The listing builds one solid part. Answer for the finished solid, in the listing's coordinates (mm). A direction names the side the tool comes from. Round coordinates to 2 decimals unless told otherwise and drop trailing zeros. Order: outer loops, then holes, each group sorted by start corner. A loop starts at its lowest first (then second) coordinate and runs counter-clockwise, first axis right, second up. Notation, with made-up numbers: (57, 20.25) - (75, 20.25) arc R5 cw to (75, 29.25) - close; hole circle Ø1 at (-23, -32). An arc over 180 degrees is marked (long way). Write item = value, one per line.
from build123d import *

# Parameters (mm, degrees)
BOSS_EXTRUDE1_DEPTH       = 10.5
BOSS_EXTRUDE2_DEPTH       = 4.5
BOSS_EXTRUDE3_DEPTH       = 7
SKETCH4_W                 = 9.5
SKETCH4_H                 = 16
BOSS_EXTRUDE4_DEPTH       = 6
SKETCH5_W                 = 2.5
SKETCH5_H                 = 2
CUT_EXTRUDE1_DEPTH        = 26.5
SKETCH6_W                 = 6
SKETCH6_H                 = 15
CUT_EXTRUDE2_DEPTH        = 5.5
F_2_CLEARANCE_HOLE1_D     = 2.5
F_2_CLEARANCE_HOLE1_DEPTH = 22
CHAMFER1_SIZE             = 0.25


with BuildPart() as part:
    # Sketch1 → Boss-Extrude1 (new body)
    with BuildSketch(Plane(origin=(0, 0, 0), x_dir=(0, -1, 0), z_dir=(-1, 0, 0))):
        with BuildLine():
            Line((14.924811557, 17.5), (-14.924811557, 17.5))
            ThreePointArc((-14.924811557, 17.5), (-16.263455967, 16.263455967), (-17.5, 14.924811557))
            Line((-17.5, 14.924811557), (-17.5, -14.924811557))
            ThreePointArc((-17.5, -14.924811557), (-16.263455967, -16.263455967), (-14.924811557, -17.5))
            Line((-14.924811557, -17.5), (14.924811557, -17.5))
            ThreePointArc((14.924811557, -17.5), (16.263455967, -16.263455967), (17.5, -14.924811557))
            Line((17.5, -14.924811557), (17.5, 14.924811557))
            ThreePointArc((17.5, 14.924811557), (16.263455967, 16.263455967), (14.924811557, 17.5))
        make_face()
    extrude(amount=-BOSS_EXTRUDE1_DEPTH)

    # Sketch2 → Boss-Extrude2 (add)
    with BuildSketch(Plane(origin=(10.5, 0, 0), x_dir=(0, 0, -1), z_dir=(1, 0, 0))):
        with BuildLine():
            Line((-17.5, -11.608186766), (-17.5, 11.608186766))
            ThreePointArc((-17.5, 11.608186766), (-14.849242405, 14.849242405), (-11.608186766, 17.5))
            Line((-11.608186766, 17.5), (11.608186766, 17.5))
            ThreePointArc((11.608186766, 17.5), (14.849242405, 14.849242405), (17.5, 11.608186766))
            Line((17.5, 11.608186766), (17.5, -11.608186766))
            ThreePointArc((17.5, -11.608186766), (14.849242405, -14.849242405), (11.608186766, -17.5))
            Line((11.608186766, -17.5), (-11.608186766, -17.5))
            ThreePointArc((-11.608186766, -17.5), (-14.849242405, -14.849242405), (-17.5, -11.608186766))
        make_face()
    extrude(amount=BOSS_EXTRUDE2_DEPTH)

    # Sketch3 → Boss-Extrude3 (add)
    with BuildSketch(Plane(origin=(15, 0, 0), x_dir=(0, 0, -1), z_dir=(1, 0, 0))):
        with BuildLine():
            Line((17.5, 14.924811557), (17.5, -14.924811557))
            ThreePointArc((17.5, -14.924811557), (16.263455967, -16.263455967), (14.924811557, -17.5))
            Line((14.924811557, -17.5), (-14.924811557, -17.5))
            ThreePointArc((-14.924811557, -17.5), (-16.263455967, -16.263455967), (-17.5, -14.924811557))
            Line((-17.5, -14.924811557), (-17.5, 14.924811557))
            ThreePointArc((-17.5, 14.924811557), (-16.263455967, 16.263455967), (-14.924811557, 17.5))
            Line((-14.924811557, 17.5), (14.924811557, 17.5))
            ThreePointArc((14.924811557, 17.5), (16.263455967, 16.263455967), (17.5, 14.924811557))
        make_face()
    extrude(amount=BOSS_EXTRUDE3_DEPTH)

    # Sketch4 → Boss-Extrude4 (add)
    with BuildSketch(Plane.XY.offset(17.5)):
        with Locations((4.75, 0)):
            Rectangle(SKETCH4_W, SKETCH4_H)
    extrude(amount=BOSS_EXTRUDE4_DEPTH)

    # Sketch5 → Cut-Extrude1 (cut, through all)
    with BuildSketch(Plane.XZ.offset(8)):
        with Locations((1.25, 22.5)):
            Rectangle(SKETCH5_W, SKETCH5_H)
    extrude(amount=-CUT_EXTRUDE1_DEPTH, mode=Mode.SUBTRACT)

    # Sketch6 → Cut-Extrude2 (cut)
    with BuildSketch(Plane.XY.offset(23.5)):
        with Locations((6, 0)):
            Rectangle(SKETCH6_W, SKETCH6_H)
    extrude(amount=-CUT_EXTRUDE2_DEPTH, mode=Mode.SUBTRACT)

    # Sketch7 → Revolve1 (revolve)
    with BuildSketch(Plane(origin=(0, 0, 0), x_dir=(-1, 0, 0), z_dir=(0, 0, -1))):
        Polygon((-32, 4.5), (-32, 0), (-22, 0), (-22, 11), (-23.5, 11), (-23.5, 2.5), (-28, 2.5), (-28, 4.5), align=None)
    revolve(axis=Axis((32, 0, 0), (-1, 0, 0)))

    # #2 Clearance Hole1
    with Locations(Plane(origin=(22, 0, 0), x_dir=(0, 0, -1), z_dir=(1, 0, 0))):
        with Locations((-13, 13), (13, 13), (13, -13), (-13, -13)):
            Hole(F_2_CLEARANCE_HOLE1_D / 2, depth=F_2_CLEARANCE_HOLE1_DEPTH)

    # Chamfer1
    chamfer1_edges = [part.edges().sort_by_distance(p)[0] for p in [
        (22, -13, 11.75),
        (0, -13, 11.75),
        (22, -13, -14.25),
        (0, -13, -14.25),
        (22, 13, -14.25),
        (0, 13, -14.25),
        (22, 13, 11.75),
        (0, 13, 11.75),
    ]]
    chamfer(chamfer1_edges, length=CHAMFER1_SIZE)


solid = part.part
Q1. Section A-A on z = 19 is taken. Determine the outline of the cut face in (x, y), then the cut area to 3 significant figures.
Model answer:
outline = (0, -8) - (9.5, -8) - (9.5, 8) - (0, 8) - close; hole (3, -7.5) - (9, -7.5) - (9, 7.5) - (3, 7.5) - close
area = 62.0 mm^2
Q2. Section C-C on y = 0 is taken. Determine the outline of the cut face in (x, z), then the cut area to 4 significant figures.
Model answer:
outline = (0, -17.5) - (22, -17.5) - (22, -11) - (23.5, -11) - (23.5, -2.5) - (28, -2.5) - (28, -4.5) - (32, -4.5) - (32, 4.5) - (28, 4.5) - (28, 2.5) - (23.5, 2.5) - (23.5, 11) - (22, 11) - (22, 17.5) - (9.5, 17.5) - (9.5, 23.5) - (9, 23.5) - (9, 18) - (3, 18) - (3, 23.5) - (2.5, 23.5) - (2.5, 21.5) - (0, 21.5) - close
area = 880.5 mm^2
Q3. Section D-D on z = 0 is taken. Determine the outline of the cut face in (x, y).
Model answer:
outline = (0, -17.5) - (22, -17.5) - (22, -11) - (23.5, -11) - (23.5, -2.5) - (28, -2.5) - (28, -4.5) - (32, -4.5) - (32, 4.5) - (28, 4.5) - (28, 2.5) - (23.5, 2.5) - (23.5, 11) - (22, 11) - (22, 17.5) - (0, 17.5) - close
Q4. For faces 5 (the face through (10.5, -15, 15)), 6 (the face through (15, -15, -15)), 7 (the face through (15, 15, -15)), 8 (the face through (1, 0, 21.5)), determine the directions among +Z, -Z, +X, -X, +Y, -Y from which every point of the face is accessible in a straight line to the end or side of a thin tool.
Model answer:
face_5 = +Z, -Y
face_6 = -Z, -Y
face_7 = -Z, +Y
face_8 = +Z, -X, +Y, -Y
Q5. Section B-B on y = -13 is taken. Determine the outline of the cut face in (x, z), then the cut area to 3 significant figures.
Model answer:
outline = (0, -17.5) - (10.5, -17.5) - (10.5, -16.49) - (15, -16.49) - (15, -17.5) - (22, -17.5) - (22, -14.5) - (21.75, -14.25) - (0.25, -14.25) - (0, -14.5) - close; (0, -11.5) - (0.25, -11.75) - (21.75, -11.75) - (22, -11.5) - (22, 11.5) - (21.75, 11.75) - (0.25, 11.75) - (0, 11.5) - close; (0, 14.5) - (0.25, 14.25) - (21.75, 14.25) - (22, 14.5) - (22, 17.5) - (15, 17.5) - (15, 16.49) - (10.5, 16.49) - (10.5, 17.5) - (0, 17.5) - close
area = 651 mm^2
Q6. Find the intervals of material crossed by line 1 (Y direction, x = 10.25, z = -13); line 2 (X direction, y = 16, z = 15); line 3 (X direction, y = 3.5, z = 20.5), in increasing order. Write a range as from..to.
Model answer:
line_1 = -17.5..-14.25, -11.75..11.75, 14.25..17.5
line_2 = 0..10.5, 15..22
line_3 = 0..3, 9..9.5
Q7. Determine the mould class of faces 1 (the face through (6, 7.5, 21)), 2 (the face through (18.451, 16.281, -16.245)), 3 (the face through (11, -17.5, 0)), 4 (the face through (0, 0, 2)) for opening direction Y: released by +Y, released by -Y, zero draft, split by the parting line, or undercut.
Model answer:
face_1 = undercut
face_2 = released by +Y
face_3 = released by -Y
face_4 = zero draft
Q8. Flat-ended cylindrical pins translate along their axes: P1, Ø3, axis at x = 5.5, y = -2.5, coming from the +Z side; P2, Ø6.5, axis at y = 13, z = 15.5, coming from the +X side; P3, Ø4.5, axis at x = 6, z = 22, coming from the +Y side; P4, Ø4, axis at x = 26.5, y = -9.5, coming from the -Z side. Find the tip coordinate at first contact, or state that the pin passes through.
Model answer:
P1 = 18
P2 = 22
P3 = 8
P4 = through
